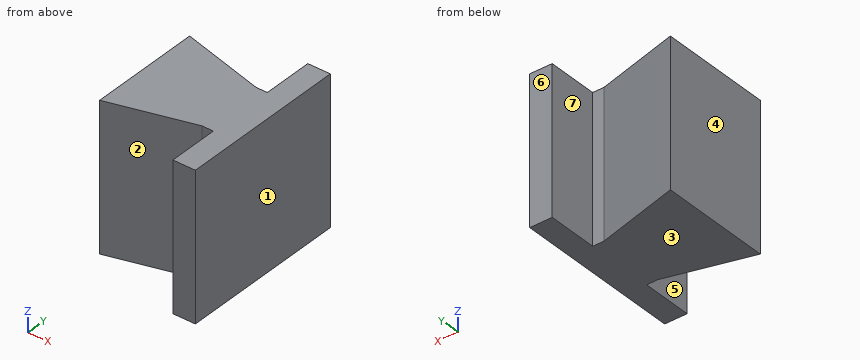
```python
from build123d import *

# Parameters (mm, degrees)
SKETCH023_W       = 10
SKETCH023_H       = 15
PAD013_DEPTH      = 13
POCKET010_DEPTH   = 13.001
POCKET010_FACE1_W = 6
POCKET010_FACE1_H = 13
PAD014_DEPTH      = 1
SKETCH026_W       = 15
SKETCH026_H       = 13
PAD015_DEPTH      = 2


with BuildPart() as part:
    # Sketch023 → Pad013 (new body)
    with BuildSketch(Plane.XY):
        with Locations((5, -7.5)):
            Rectangle(SKETCH023_W, SKETCH023_H)
    extrude(amount=PAD013_DEPTH)

    # Sketch025 (on Face6 of Pad013) → Pocket010 (cut, through all)
    with BuildSketch(Plane.XY.offset(13)):
        Polygon((10, -4.5), (2.5, -2.5), (2.5, -12.5), (10, -10.5), (10, -15), (0, -15), (0, 0), (10, 0), align=None)
    extrude(amount=-POCKET010_DEPTH, mode=Mode.SUBTRACT)

    # Pocket010 Face1 → Pad014 (add)
    with BuildSketch(Plane(origin=(10, -7.5, 6.5), x_dir=(0, -1, 0), z_dir=(1, 0, 0))):
        Rectangle(POCKET010_FACE1_W, POCKET010_FACE1_H)
    extrude(amount=PAD014_DEPTH)

    # Sketch026 (on Face6 of Pad014) → Pad015 (join)
    with BuildSketch(Plane.YZ.offset(11)):
        with Locations((-7.5, 6.5)):
            Rectangle(SKETCH026_W, SKETCH026_H)
    extrude(amount=PAD015_DEPTH)


with BuildPart() as part_1:
    # Body004 placement: moved
    add(part.part.moved(Location((0, 0, 16))))


solid = part_1.part
```
The listing builds one solid part. Answer for the finished solid, in the listing's coordinates (mm). Face numbers are marked on the shaded views. A direction names the side the tool comes from. Coordinates: 2 decimals unless noted, no trailing zeros. Loops run counter-clockwise (first coordinate to the right, second up) from the corner with the lowest first, then second, coordinate; pieces in that order, holes last. Notation, with made-up numbers: (64.5, 80.5) - (101.5, 80.5) arc R26 cw to (101.5, 115.5) - close; hole circle Ø3 at (5.5, 60). An arc over 180 degrees is marked (long way). Write item = value, one per line.
1) Which of the six approach directions +Z, -Z, +X, -X, +Y, -Y give full straight-line access (tool end or side, diameter ignored) to the marked faces 5, 6 and 7?
Responses:
face_5 = +Z, -Z, -Y
face_6 = +Z, -Z, +X, -X, +Y
face_7 = +Z, -Z, +Y
2) Find the intervals of material crossed by line 1 along X through (y, z) = (-1.75, 19.5); line 2 along Y through (x, z) = (6.75, 27.5); line 3 along Y through (x, z) = (4, 19.5), in increasing order.
Responses:
line_1 = 11 to 13
line_2 = -11.37 to -3.63
line_3 = -12.1 to -2.9
3) Section B-B (y = -2.25) is taken. Determine the outline of the cut face in (x, z).
Responses:
outline = (11, 16) - (13, 16) - (13, 29) - (11, 29) - close
4) Determine the mould class of the marked faces 1, 2, 3 and 4 for opening direction X: pulls with the +X half, pulls with the -X half, needs draft (parallel to the pull), parting line crosses it, or undercut.
Responses:
face_1 = pulls with the +X half
face_2 = undercut
face_3 = needs draft
face_4 = pulls with the -X half
5) Section C-C (x = 10.5) is taken. Determine the outline of the cut face in (y, z), plus the area to 3 significant figures.
Responses:
outline = (-10.5, 16) - (-4.5, 16) - (-4.5, 29) - (-10.5, 29) - close
area = 78.0 mm^2
6) Each of these flat-tipped pins is pushed along its axis until it touches: P1, Ø6, axis at x = 6, z = 22.5, coming from the -Y side; P2, Ø4, axis at x = 5, z = 27.5, coming from the +Y side; P3, Ø1.5, axis at x = 9, z = 25.5, coming from the +Y side. Where does it stop, or does it pass through?
Responses:
P1 = -12.37
P2 = -2.63
P3 = -4.03
7) Section A-A (z = 21.75) is taken. Determine the outline of the cut face in (x, y), plus the area to 3 significant figures.
Responses:
outline = (2.5, -12.5) - (10, -10.5) - (11, -10.5) - (11, -15) - (13, -15) - (13, 0) - (11, 0) - (11, -4.5) - (10, -4.5) - (2.5, -2.5) - close
area = 96.0 mm^2
